from build123d import *

# Parameters (mm, degrees)
F0_R     = 2
F0_R_2   = 5
F1_DEPTH = 6


with BuildPart() as f1:
    # F0 (on Top) → F1 (new body)
    with BuildSketch(Plane.XY):
        with BuildLine():
            Line((1.422636, 15.288272), (1.598278, 17.175797))
            ThreePointArc((1.598278, 17.175797), (0, 18.85), (-1.598278, 17.175797))
            Line((-1.598278, 17.175797), (-1.422236, 15.28397))
            ThreePointArc((-1.422236, 15.28397), (-1.633511, 14.531637), (-2.321448, 14.160981))
            ThreePointArc((-2.321448, 14.160981), (-2.983533, 14.036418), (-3.639042, 13.880918))
            ThreePointArc((-3.639042, 13.880918), (-4.420263, 13.940625), (-4.918657, 14.54517))
            Line((-4.918657, 14.54517), (-5.525926, 16.34095))
            ThreePointArc((-5.525926, 16.34095), (-7.666986, 17.220332), (-8.446126, 15.040793))
            Line((-8.446126, 15.040793), (-7.515828, 13.384126))
            ThreePointArc((-7.515828, 13.384126), (-7.402836, 12.610902), (-7.880538, 11.992482))
            ThreePointArc((-7.880538, 11.992482), (-8.434718, 11.609394), (-8.970308, 11.200718))
            ThreePointArc((-8.970308, 11.200718), (-9.708274, 10.937512), (-10.40947, 11.287075))
            Line((-10.40947, 11.287075), (-11.694648, 12.680604))
            ThreePointArc((-11.694648, 12.680604), (-14.00828, 12.613112), (-13.833562, 10.305099))
            Line((-13.833562, 10.305099), (-12.309865, 9.170045))
            ThreePointArc((-12.309865, 9.170045), (-11.892143, 8.509628), (-12.077011, 7.750374))
            ThreePointArc((-12.077011, 7.750374), (-12.427465, 7.175), (-12.750526, 6.583812))
            ThreePointArc((-12.750526, 6.583812), (-13.317637, 6.043204), (-14.100392, 6.077343))
            Line((-14.100392, 6.077343), (-15.841259, 6.827666))
            ThreePointArc((-15.841259, 6.827666), (-17.927415, 5.82497), (-16.829049, 3.78756))
            Line((-16.829049, 3.78756), (-14.975415, 3.37038))
            ThreePointArc((-14.975415, 3.37038), (-14.32519, 2.936961), (-14.18526, 2.168156))
            ThreePointArc((-14.18526, 2.168156), (-14.271389, 1.499983), (-14.326063, 0.828505))
            ThreePointArc((-14.326063, 0.828505), (-14.624259, 0.103971), (-15.353227, -0.183216))
            Line((-15.353227, -0.183216), (-17.248772, -0.205837))
            ThreePointArc((-17.248772, -0.205837), (-18.746738, -1.970362), (-16.914641, -3.384883))
            Line((-16.914641, -3.384883), (-15.051579, -3.012055))
            ThreePointArc((-15.051579, -3.012055), (-14.281282, -3.143532), (-13.840748, -3.788956))
            ThreePointArc((-13.840748, -3.788956), (-13.647661, -4.434394), (-13.424493, -5.070058))
            ThreePointArc((-13.424493, -5.070058), (-13.402214, -5.85324), (-13.95135, -6.412097))
            Line((-13.95135, -6.412097), (-15.673816, -7.203749))
            ThreePointArc((-15.673816, -7.203749), (-16.324579, -9.425), (-14.075537, -9.972048))
            Line((-14.075537, -9.972048), (-12.525188, -8.873678))
            ThreePointArc((-12.525188, -8.873678), (-11.768011, -8.68048), (-11.103045, -9.090923))
            ThreePointArc((-11.103045, -9.090923), (-10.664128, -9.602024), (-10.201706, -10.091961))
            ThreePointArc((-10.201706, -10.091961), (-9.862804, -10.798372), (-10.137158, -11.532267))
            Line((-10.137158, -11.532267), (-11.388715, -12.956067))
            ThreePointArc((-11.388715, -12.956067), (-11.079752, -15.24997), (-8.802646, -14.834956))
            Line((-8.802646, -14.834956), (-7.833079, -13.200961))
            ThreePointArc((-7.833079, -13.200961), (-7.219944, -12.716495), (-6.445525, -12.820987))
            ThreePointArc((-6.445525, -12.820987), (-5.836671, -13.109377), (-5.214952, -13.368873))
            ThreePointArc((-5.214952, -13.368873), (-4.618026, -13.876368), (-4.570159, -14.658404))
            Line((-4.570159, -14.658404), (-5.134401, -16.468164))
            ThreePointArc((-5.134401, -16.468164), (-3.919135, -18.438082), (-2.007697, -17.132765))
            Line((-2.007697, -17.132765), (-1.786559, -15.245678))
            ThreePointArc((-1.786559, -15.245678), (-1.423482, -14.553712), (-0.673515, -14.334186))
            ThreePointArc((-0.673515, -14.334186), (0, -14.35), (0.673515, -14.334186))
            ThreePointArc((0.673515, -14.334186), (1.42525, -14.555013), (1.787062, -15.249969))
            Line((1.787062, -15.249969), (2.007697, -17.132765))
            ThreePointArc((2.007697, -17.132765), (3.919135, -18.438082), (5.134401, -16.468164))
            Line((5.134401, -16.468164), (4.568873, -14.654279))
            ThreePointArc((4.568873, -14.654279), (4.619112, -13.87446), (5.214952, -13.368873))
            ThreePointArc((5.214952, -13.368873), (5.836671, -13.109377), (6.445525, -12.820987))
            ThreePointArc((6.445525, -12.820987), (7.222088, -12.716965), (7.835284, -13.204676))
            Line((7.835284, -13.204676), (8.802646, -14.834956))
            ThreePointArc((8.802646, -14.834956), (11.079752, -15.24997), (11.388715, -12.956067))
            Line((11.388715, -12.956067), (10.134305, -11.529022))
            ThreePointArc((10.134305, -11.529022), (9.86302, -10.796187), (10.201706, -10.091961))
            ThreePointArc((10.201706, -10.091961), (10.664128, -9.602024), (11.103045, -9.090923))
            ThreePointArc((11.103045, -9.090923), (11.770162, -8.680038), (12.528714, -8.876175))
            Line((12.528714, -8.876175), (14.075537, -9.972048))
            ThreePointArc((14.075537, -9.972048), (16.324579, -9.425), (15.673816, -7.203749))
            Line((15.673816, -7.203749), (13.947425, -6.410292))
            ThreePointArc((13.947425, -6.410292), (13.401522, -5.851156), (13.424493, -5.070058))
            ThreePointArc((13.424493, -5.070058), (13.647661, -4.434394), (13.840748, -3.788956))
            ThreePointArc((13.840748, -3.788956), (14.283067, -3.142253), (15.055815, -3.012903))
            Line((15.055815, -3.012903), (16.914641, -3.384883))
            ThreePointArc((16.914641, -3.384883), (18.746738, -1.970362), (17.248772, -0.205837))
            Line((17.248772, -0.205837), (15.348907, -0.183165))
            ThreePointArc((15.348907, -0.183165), (14.622779, 0.105593), (14.326063, 0.828505))
            ThreePointArc((14.326063, 0.828505), (14.271389, 1.499983), (14.18526, 2.168156))
            ThreePointArc((14.18526, 2.168156), (14.3263, 2.938856), (14.979629, 3.371328))
            Line((14.979629, 3.371328), (16.829049, 3.78756))
            ThreePointArc((16.829049, 3.78756), (17.927415, 5.82497), (15.841259, 6.827666))
            Line((15.841259, 6.827666), (14.096424, 6.075633))
            ThreePointArc((14.096424, 6.075633), (13.315625, 6.044084), (12.750526, 6.583812))
            ThreePointArc((12.750526, 6.583812), (12.427465, 7.175), (12.077011, 7.750374))
            ThreePointArc((12.077011, 7.750374), (11.892386, 8.51181), (12.31333, 9.172626))
            Line((12.31333, 9.172626), (13.833562, 10.305099))
            ThreePointArc((13.833562, 10.305099), (14.00828, 12.613112), (11.694648, 12.680604))
            Line((11.694648, 12.680604), (10.406542, 11.2839))
            ThreePointArc((10.406542, 11.2839), (9.706078, 10.937498), (8.970308, 11.200718))
            ThreePointArc((8.970308, 11.200718), (8.434718, 11.609394), (7.880538, 11.992482))
            ThreePointArc((7.880538, 11.992482), (7.402171, 12.612994), (7.517943, 13.387893))
            Line((7.517943, 13.387893), (8.446126, 15.040793))
            ThreePointArc((8.446126, 15.040793), (7.666986, 17.220332), (5.525926, 16.34095))
            Line((5.525926, 16.34095), (4.917273, 14.541077))
            ThreePointArc((4.917273, 14.541077), (4.418263, 13.939719), (3.639042, 13.880918))
            ThreePointArc((3.639042, 13.880918), (2.983533, 14.036418), (2.321448, 14.160981))
            ThreePointArc((2.321448, 14.160981), (1.632052, 14.533278), (1.422636, 15.288272))
        make_face()
        with Locations((-10.116822, -0.941412)):
            Circle(F0_R, mode=Mode.SUBTRACT)
        with Locations((-6.487995, -7.819352)):
            Circle(F0_R, mode=Mode.SUBTRACT)
        with Locations((0.941412, -10.116822)):
            Circle(F0_R, mode=Mode.SUBTRACT)
        with Locations((7.819352, -6.487995)):
            Circle(F0_R, mode=Mode.SUBTRACT)
        Circle(F0_R_2, mode=Mode.SUBTRACT)
        with Locations((-7.819352, 6.487995)):
            Circle(F0_R, mode=Mode.SUBTRACT)
        with Locations((-0.941412, 10.116822)):
            Circle(F0_R, mode=Mode.SUBTRACT)
        with Locations((6.487995, 7.819352)):
            Circle(F0_R, mode=Mode.SUBTRACT)
        with Locations((10.116822, 0.941412)):
            Circle(F0_R, mode=Mode.SUBTRACT)
    extrude(amount=F1_DEPTH)


solid = f1.part
Design review of the part built by this model. Coordinates are the model's own, in mm. A direction names the side the tool comes from. Round coordinates to 2 decimals unless told otherwise and drop trailing zeros. Write each loop counter-clockwise with the first axis right and the second up, starting at its lowest first coordinate (ties: lowest second). Pieces come first, ordered by that corner, then holes. Notation, with made-up numbers: M 75,74 L 131,74 A18 ccw 131,79 Z; hole C -7.5,-32 d9. An arc over 180 degrees is marked long. One line per item, written item: value. Start each with the question number.
1. Draft analysis for pull direction X (two halves, no side actions). For faces 1 (the face through (-13.082, 9.746, 2.958)), 2 (the face through (-10.67, -9.595, 2.958)), 3 (the face through (-8.427, 11.615, 2.958)), 4 (the face through (13.645, -4.443, 2.958)), state which applies: pulls with the +X half, pulls with the -X half, needs draft (parallel to the pull), parting line crosses it, or undercut.
2. For faces 5 (the face through (-1.51, 16.24, 2.96)), 6 (the face through (-14.8, -6.8, 3)), 7 (the face through (11.06, 11.99, 2.96)), list the 3-axis set-ups (+Z, -Z, +X, -X, +Y, -Y) from which the entire face can be reached by the end or side of a thin tool; tool diameter is ignored.
3. Clearance check with flat-ended pins moving along their axes: P1, Ø2, axis at x = 15, z = 2.5, coming from the -Y side (3 decimals); P2, Ø2.5, axis at x = 10.12, y = 0.94, coming from the -Z side; P3, Ø2, axis at x = 10, z = 4, coming from the +Y side; P4, Ø1.5, axis at x = -2.5, z = 1.5, coming from the -Y side. State where each tip first meets the part, or that it passes through.
4. Take a section at B-B on x = 0. State the section outline as (y, z) points, then the cut area to 4 significant figures.
5. Take a section at A-A on y = -2.5. State the section outline as (x, z) points, then the cut area to 3 significant figures.
6. Take a section at C-C on z = 4.25. State how many separate pieces and enclosed holes the cut face has, then the cut area to 3 significant figures.
7. To check wall thickness, follow probe 1 along Y at (x, z) = (-15.5, 3.7); probe 2 along X at (y, z) = (-9, 2.9); probe 3 along Y at (x, z) = (-7, 3.9). State the ranges of each line that lie inside material, in increasing order. Write a range as from..to.
Computed:
1. face 1: pulls with the -X half
1. face 2: undercut
1. face 3: undercut
1. face 4: pulls with the +X half
2. face 5: +Z, -Z
2. face 6: +Z, -Z, -X
2. face 7: +Z, -Z, +Y
3. P1: stops at y = -10.225
3. P2: passes through
3. P3: stops at y = 11.93
3. P4: stops at y = -18.44
4. outline: M -14.35,0 L -11.88,0 L -11.88,6 L -14.35,6 Z; M -8.35,0 L -5,0 L -5,6 L -8.35,6 Z; M 5,0 L 8.35,0 L 8.35,6 L 5,6 Z; M 11.88,0 L 18.85,0 L 18.85,6 L 11.88,6 Z
4. area: 96.85 mm²
5. outline: M -18.6,0 L -11.37,0 L -11.37,6 L -18.6,6 Z; M -8.86,0 L -4.33,0 L -4.33,6 L -8.86,6 Z; M 4.33,0 L 18.6,0 L 18.6,6 L 4.33,6 Z
5. area: 156 mm²
6. separate pieces: 1
6. enclosed holes: 9
6. area: 663 mm²
7. probe 1: y = -10.12..-7.12, -3.1..-0.18, 3.49..6.68
7. probe 2: x = -16.49..-12.7, -11.18..-8.1, -4.87..-0.72, 2.6..11.18, 12.7..16.49
7. probe 3: y = -12.68..-9.75, -5.89..4.66, 8.31..17.36
